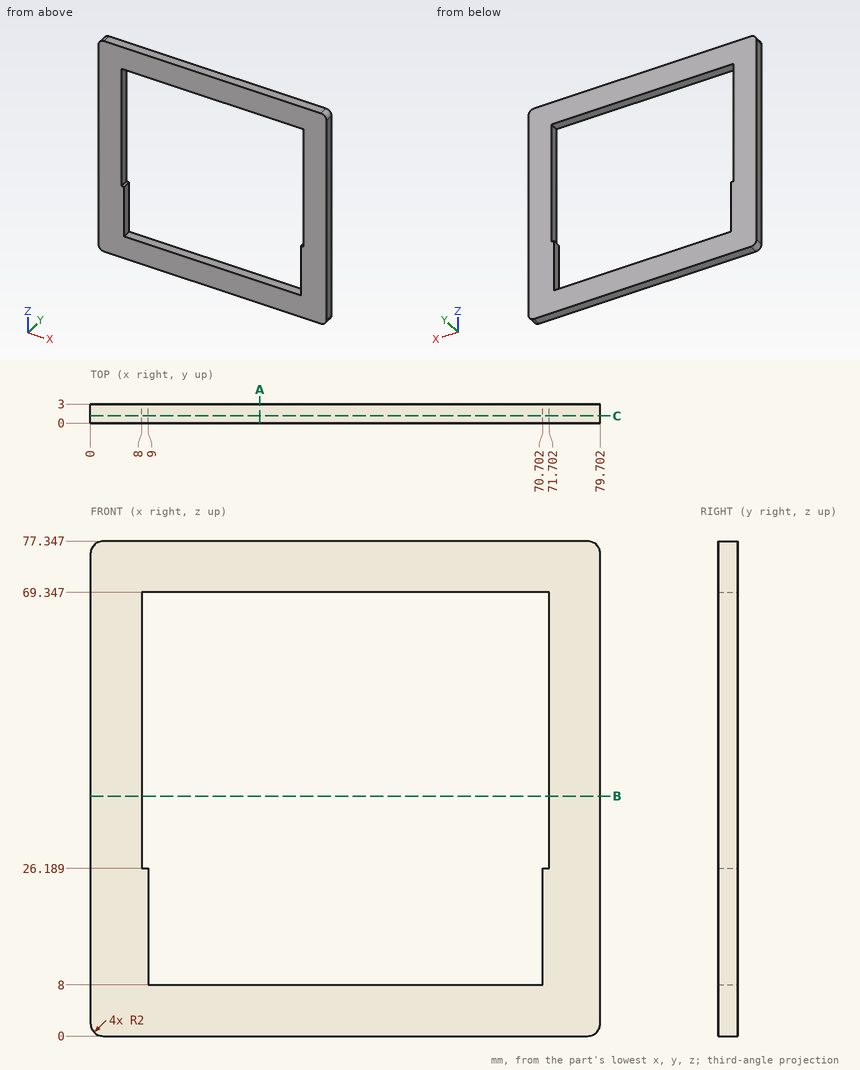
Could you check a few things on this drawing? It's one solid part, dimensions in mm from its lowest x, y, z. Coordinates: 2 decimals unless noted, no trailing zeros. Order: outer loops, then holes, each group sorted by start corner. A loop starts at its lowest first (then second) coordinate and runs counter-clockwise, first axis right, second up. Notation, with made-up numbers: (65.25, 5) - (118.25, 5) arc R18 cw to (118.25, 11) - close; hole circle Ø2 at (58.5, 20). An arc over 180 degrees is marked (long way). One line per question, with ' | ' between items. Start each with the question number.
1. If we section it at A-A (x = 26.5): Write out the boundary of the cut face in (y, z), and give its area (3 significant figures).
2. If we section it at B-B (z = 37.5): Write out the boundary of the cut face in (x, y), and give its area (3 significant figures).
3. If we section it at C-C (y = 1.15): Write out the boundary of the cut face in (x, z).
4. I'm going to push flat-ended pins straight in: pin 1 Ø12 at (x, z) = (56.5, 62) entering from -Y; pin 2 Ø1.5 at (y, z) = (1, 18.5) entering from -X. Where does each tip first touch, or does it pass through?
5. Please list where these lines run through material, in increasing order: line 1 along Z through (x, y) = (12, 2.4); line 2 along Z through (x, y) = (71.5, 2.5); line 3 along X through (y, z) = (0.5, 56.5). Write a range as [from, to].
Model answer:
1) outline: (0, 0) - (3, 0) - (3, 8) - (0, 8) - close; (0, 69.35) - (3, 69.35) - (3, 77.35) - (0, 77.35) - close | area: 48.0 mm²
2) outline: (0, 0) - (8, 0) - (8, 3) - (0, 3) - close; (71.7, 0) - (79.7, 0) - (79.7, 3) - (71.7, 3) - close | area: 48.0 mm²
3) outline: (0, 2) arc R2 ccw to (2, 0) - (77.7, 0) arc R2 ccw to (79.7, 2) - (79.7, 75.35) arc R2 ccw to (77.7, 77.35) - (2, 77.35) arc R2 ccw to (0, 75.35) - close; hole (8, 26.19) - (9, 26.19) - (9, 8) - (70.7, 8) - (70.7, 26.19) - (71.7, 26.19) - (71.7, 69.35) - (8, 69.35) - close
4) pin 1: passes through | pin 2: stops at x = 0
5) line 1: z = [0, 8], [69.35, 77.35] | line 2: z = [0, 26.19], [69.35, 77.35] | line 3: x = [0, 8], [71.7, 79.7]
